Autodesk Inventor part; units mm, degrees
ref_plane "YZ Plane" through (0, 0, 0) normal (1, 0, 0) x (0, 1, 0)
ref_plane "XZ Plane" through (0, 0, 0) normal (0, 1, 0) x (-1, 0, 0)
ref_plane "XY Plane" through (0, 0, 0) normal (0, 0, 1) x (1, 0, 0)
sketch "Sketch1" plane through (0, 0, 0) normal (0, 1, 0) x (-1, 0, 0)
  line L0 (-348.8673, 325.8519) -> (-348.8673, -174.1481)
  line L1 (1.1327, -174.1481) -> (1.1327, 325.8519)
  line L2 (-98.8673, -174.1481) -> (-98.8673, -204.1481)
  line L3 (-58.8673, -203.2202) -> (-58.8673, -174.1481)
  line L4 (-128.8673, -204.1481) -> (-128.8673, -234.1481)
  line L5 (-128.8673, -234.1481) -> (-28.8673, -234.1481)
  line L6 (-28.8673, -234.1481) -> (-28.8673, -203.2202)
  line L7 (-58.8673, -174.1481) -> (1.1327, -174.1481)
  line L8 (-28.8673, -203.2202) -> (-58.8673, -203.2202)
  line L9 (-98.8673, -204.1481) -> (-128.8673, -204.1481)
  line L10 (-99.6673, 325.8519) -> (-99.6673, 296.2519)
  line L11 (-59.2673, 296.2519) -> (-59.2673, 325.8519)
  line L12 (-130.0673, 296.2519) -> (-130.0673, 265.4519)
  line L13 (-130.0673, 265.4519) -> (-28.8673, 265.4519)
  line L14 (-28.8673, 265.4519) -> (-28.8673, 296.2519)
  line L15 (-28.8673, 296.2519) -> (-59.2673, 296.2519)
  line L16 (-99.6673, 296.2519) -> (-130.0673, 296.2519)
  line L17 (1.1327, 325.8519) -> (-59.2673, 325.8519)
  line L18 (-320.4673, 296.2519) -> (-320.4673, 265.4519)
  line L19 (-320.4673, 265.4519) -> (-219.2673, 265.4519)
  line L20 (-219.2673, 265.4519) -> (-219.2673, 296.2519)
  line L21 (-290.0673, 325.8519) -> (-290.0673, 296.2519)
  line L22 (-249.6673, 296.2519) -> (-249.6673, 325.8519)
  line L23 (-318.8673, -204.1481) -> (-318.8673, -234.1481)
  line L24 (-318.8673, -234.1481) -> (-218.8673, -234.1481)
  line L25 (-218.8673, -234.1481) -> (-218.8673, -204.1481)
  line L26 (-288.8673, -174.1481) -> (-288.8673, -204.1481)
  line L27 (-248.8673, -204.1481) -> (-248.8673, -174.1481)
  line L28 (-99.6673, 325.8519) -> (-249.6673, 325.8519)
  line L29 (-290.0673, 325.8519) -> (-348.8673, 325.8519)
  line L30 (-219.2673, 296.2519) -> (-249.6673, 296.2519)
  line L31 (-290.0673, 296.2519) -> (-320.4673, 296.2519)
  line L32 (-348.8673, -174.1481) -> (-288.8673, -174.1481)
  line L33 (-248.8673, -174.1481) -> (-98.8673, -174.1481)
  line L34 (-218.8673, -204.1481) -> (-248.8673, -204.1481)
  line L35 (-288.8673, -204.1481) -> (-318.8673, -204.1481)
  point P0 (0, 0)
  dimension "d0" = 500
  dimension "d1" = 350
  dimension "d5" = 100
  dimension "d6" = 40.4
  dimension "d7" = 40
  dimension "d8" = 30
  dimension "d9" = 30.4
  dimension "d11" = 30
  dimension "d15" = 30
  dimension "d20" = 30
  dimension "d30" = 500
  dimension "d33" = 40.4
  dimension "d35" = 30.4
  dimension "d36" = 29.6
  dimension "d37" = 29.6
  dimension "d38" = 30.8
  dimension "d39" = 30.4
  dimension "d40" = 30.4
  dimension "d41" = 30.8
  dimension "d42" = 30.8
  dimension "d43" = 29.6
extrude "Extrusion2" add sketch "Sketch1" against normal blind 3
properties part number "TopCoverLayer" material "Acrylic"
CAD build for the part. Positions are in the model's coordinates, mm. Give positions to 0.01 mm unless a question says otherwise; leave off trailing zeros. Order: outer loops, then holes, each group sorted by start corner. A loop starts at its lowest first (then second) coordinate and runs counter-clockwise, first axis right, second up. Notation, with made-up numbers: M 63,81 L 117,81 A21 cw 117,95 Z; hole C 85,22 d2. An arc over 180 degrees is marked long. Put each result on its own line as item: value. Start each with the question number.
(1) Flat gauge pins, fed straight in: pin 1 Ø0.9 at (y, z) = (-1, -186) entering from +X; pin 2 Ø1 at (x, y) = (165.5, -2) entering from -Z; pin 3 Ø1 at (x, z) = (129, 52) entering from +Y; pin 4 Ø1.5 at (y, z) = (-1.5, -226.5) entering from +X. Where does each tip first touch, or does it go through?
(2) Drill centre lines: line 1 along Z through (x, y) = (305, -2); line 2 along Z through (x, y) = (45, -1.3); line 3 along X through (y, z) = (-1.25, 269). Where is each one in solid material? Low to high.
(3) Saw through at C-C, the plane x = 276. Write the cut outline in (y, z).
(4) Saw through at A-A, the plane z = 286.5. Write the cut outline in (x, y).
(5) Saw through at B-B, the plane x = 236. Write the cut outline in (y, z).
Check result:
1. pin 1: stops at x = 288.87
1. pin 2: stops at z = -174.15
1. pin 3: stops at y = 0
1. pin 4: stops at x = 318.87
2. line 1: z = -234.15 to -204.15, -174.15 to 265.45, 296.25 to 325.85
2. line 2: z = -234.15 to -203.22, -174.15 to 265.45, 296.25 to 325.85
2. line 3: x = -1.13 to 28.87, 130.07 to 219.27, 320.47 to 348.87
3. outline: M -3,-234.15 L 0,-234.15 L 0,265.45 L -3,265.45 Z
4. outline: M -1.13,-3 L 28.87,-3 L 28.87,0 L -1.13,0 Z; M 130.07,-3 L 219.27,-3 L 219.27,0 L 130.07,0 Z; M 320.47,-3 L 348.87,-3 L 348.87,0 L 320.47,0 Z
5. outline: M -3,-234.15 L 0,-234.15 L 0,-204.15 L -3,-204.15 Z; M -3,-174.15 L 0,-174.15 L 0,265.45 L -3,265.45 Z; M -3,296.25 L 0,296.25 L 0,325.85 L -3,325.85 Z
